Design review of the part built by this model. Coordinates are the model's own, in mm. Coordinates: 2 decimals unless noted, no trailing zeros. Loops run counter-clockwise (first coordinate to the right, second up) from the corner with the lowest first, then second, coordinate; pieces in that order, holes last. Notation, with made-up numbers: (-23.5, -27.5) -> (27.5, -27.5) arc R11 ccw to (27.5, -18.5) -> close; hole circle Ø9 at (0, 8.25). An arc over 180 degrees is marked (long way). Answer in a Markdown table with one row per item.
Autodesk Inventor part; units mm, degrees
ref_plane "Start plane" through (0, 0, -17.5) normal (0, 0, 1) x (1, 0, 0)
ref_plane "End plane" through (0, 0, 447.5) normal (0, 0, 1) x (1, 0, 0)
ref_plane "Work Plane4" through (17.5, 0, 447.5) normal (-0.7071, 0, 0.7071) x (0.7071, 0, 0.7071)
ref_plane "Start plane" through (0, 0, -17.5) normal (0, 0, 1) x (1, 0, 0)
ref_plane "End plane" through (0, 0, 447.5) normal (0, 0, 1) x (1, 0, 0)
sketch "Sketch" plane through (0, 0, 0) normal (0, 0, 1) x (1, 0, 0)
  line L0 (-17.5, -14.3) -> (-17.5, 14.3)
  line L1 (-14.3, 17.5) -> (14.3, 17.5)
  line L2 (17.5, 14.3) -> (17.5, -14.3)
  line L3 (14.3, -17.5) -> (-14.3, -17.5)
  arc A0 (-17.5, -14.3) -> (-14.3, -17.5) centre (-14.3, -14.3) ccw
  arc A1 (-14.3, 17.5) -> (-17.5, 14.3) centre (-14.3, 14.3) ccw
  arc A2 (17.5, 14.3) -> (14.3, 17.5) centre (14.3, 14.3) ccw
  arc A3 (14.3, -17.5) -> (17.5, -14.3) centre (14.3, -14.3) ccw
  arc A4 (-14.3, 15.9) -> (-15.9, 14.3) centre (-14.3, 14.3) ccw
  line L4 (-14.3, 15.9) -> (14.3, 15.9)
  arc A5 (15.9, 14.3) -> (14.3, 15.9) centre (14.3, 14.3) ccw
  line L5 (15.9, 14.3) -> (15.9, -14.3)
  arc A6 (14.3, -15.9) -> (15.9, -14.3) centre (14.3, -14.3) ccw
  line L6 (14.3, -15.9) -> (-14.3, -15.9)
  arc A7 (-15.9, -14.3) -> (-14.3, -15.9) centre (-14.3, -14.3) ccw
  line L7 (-15.9, -14.3) -> (-15.9, 14.3)
  line L8 (0, 25.4278) -> (0, -25.4278) construction
  line L9 (-25.4278, 0) -> (25.4278, 0) construction
  dimension "d7" = 3.2
  dimension "d10" = 35
  dimension "d11" = 35
  dimension "d12" = 1.6
  dimension "d15" = 17.5
  dimension "d16" = 17.5
extrude "Body" add sketch "Sketch" along normal up to surface (465 mm away) from surface at -17.5
sketch "Sketch3" plane through (0, 0, 0) normal (0, 0, 1) x (1, 0, 0)
  line L0 (0, 0) -> (10, 0)
ref_plane "Work Plane3" through (0, 0, 0) normal (0, -1, 0) x (1, 0, 0)
sketch "Sketch4" plane through (0, 0, 0) normal (0, -1, 0) x (1, 0, 0)
  line L0 (-2, -17.5) -> (12, -17.5)
  line L1 (-2, 447.5) -> (12, 447.5)
  dimension "d18" = 465
ref_plane "Work Plane4" through (17.5, 0, 447.5) normal (-0.7071, 0, 0.7071) x (0.7071, 0, 0.7071)
split "Split1" plane through (17.5, 0, 447.5) removes the side toward (-0.7071, 0, 0.7071)
ref_plane "Work Plane5" through (17.5, 0, -17.5) normal (-0.7071, 0, -0.7071) x (-0.7071, 0, 0.7071)
split "Split2" plane through (17.5, 0, -17.5) removes the side toward (-0.7071, 0, -0.7071)
ref_plane "Work Plane6" through (-730, 0, 215) normal (1, 0, 0) x (0, 0, -1)
ref_plane "Work Plane7" through (0, 0, 215) normal (1, 0, 0) x (0, 0, -1)
ref_plane "Work Plane8" through (-365, 0, 215) normal (1, 0, 0) x (0, 0, -1)
sketch "Sketch5" plane through (-365, 0, 215) normal (1, 0, 0) x (0, 0, -1)
  arc A0 (-17.5, -11.5) -> (-11.5, -17.5) centre (-11.5, -11.5) ccw
  line L0 (-17.5, -11.5) -> (-17.5, 11.5)
  arc A1 (-11.5, 17.5) -> (-17.5, 11.5) centre (-11.5, 11.5) ccw
  line L1 (-11.5, 17.5) -> (11.5, 17.5)
  arc A2 (17.5, 11.5) -> (11.5, 17.5) centre (11.5, 11.5) ccw
  line L2 (17.5, 11.5) -> (17.5, -11.5)
  arc A3 (11.5, -17.5) -> (17.5, -11.5) centre (11.5, -11.5) ccw
  line L3 (11.5, -17.5) -> (-11.5, -17.5)
  arc A4 (-11.5, 14.5) -> (-14.5, 11.5) centre (-11.5, 11.5) ccw
  line L4 (-11.5, 14.5) -> (11.5, 14.5)
  arc A5 (14.5, 11.5) -> (11.5, 14.5) centre (11.5, 11.5) ccw
  line L5 (14.5, 11.5) -> (14.5, -11.5)
  arc A6 (11.5, -14.5) -> (14.5, -11.5) centre (11.5, -11.5) ccw
  line L6 (11.5, -14.5) -> (-11.5, -14.5)
  arc A7 (-14.5, -11.5) -> (-11.5, -14.5) centre (-11.5, -11.5) ccw
  line L7 (-14.5, -11.5) -> (-14.5, 11.5)
extrude "Extrusion2" cut sketch "Sketch5" along normal up to surface (730 mm away) from surface at -365 contours L0 A1 L1 A2 L2 A3 L3 A0 | L4 A5 L5 A6 L6 A7 L7 A4
equation "\"d7\" = G_IR"
equation "\"d10\" = G_H"
equation "\"d11\" = G_W"
equation "\"d12\" = G_T"
equation "\"d15\" = 0.5 * d10"
equation "\"d16\" = 0.5 * d11"
equation "\"d3\" = G_L"
equation "\"G_W\" = 35"
equation "\"G_H\" = 35"
equation "\"G_T\" = 1.6"
equation "\"G_IR\" = 3.2"
equation "\"G_L\" = d18"
equation "\"G_OFFSET_START\" = 17.5"
equation "\"G_OFFSET_END\" = 17.5"
equation "\"d13\" = -G_OFFSET_START"
equation "\"d14\" = G_OFFSET_END + B_L"
properties part number "AS C350L0 35x35x3.0 SHS 00000050" material "Steel, Mild"
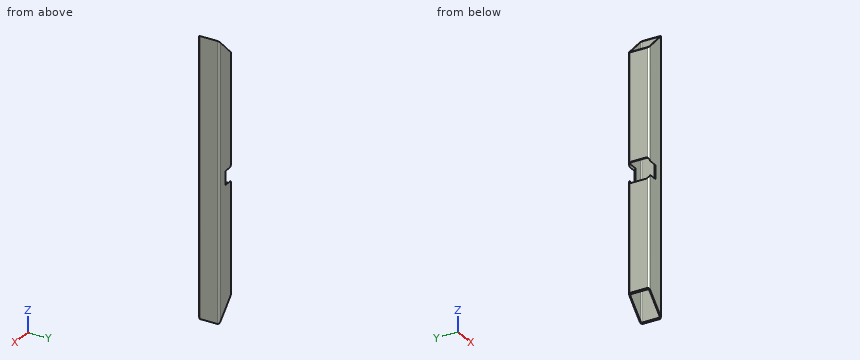
(1) Take a section at C-C on z = 144.5. Give the boundary of the cut face in (x, y).
Evaluation:
| item | result |
|---|---|
| outline | (-17.5, -14.3) arc R3.2 ccw to (-14.3, -17.5) -> (14.3, -17.5) arc R3.2 ccw to (17.5, -14.3) -> (17.5, 14.3) arc R3.2 ccw to (14.3, 17.5) -> (-14.3, 17.5) arc R3.2 ccw to (-17.5, 14.3) -> close; hole (-15.9, -14.3) arc R1.6 ccw to (-14.3, -15.9) -> (14.3, -15.9) arc R1.6 ccw to (15.9, -14.3) -> (15.9, 14.3) arc R1.6 ccw to (14.3, 15.9) -> (-14.3, 15.9) arc R1.6 ccw to (-15.9, 14.3) -> close |
(2) Take a section at A-A on x = 7.5. Give the boundary of the cut face in (y, z), and give its area (3 significant figures).
Evaluation:
| item | result |
|---|---|
| outline | (-17.5, -7.5) -> (-15.9, -7.5) -> (-15.9, 437.5) -> (-17.5, 437.5) -> close; (15.9, -7.5) -> (17.5, -7.5) -> (17.5, 437.5) -> (15.9, 437.5) -> close |
| area | 1,420 mm² |
(3) For pin 1 (10 mm diameter, centred on x = 13, y = 4.5, fed in from +Z); pin 2 (1.3 mm diameter, centred on y = -17, z = 207.5, fed in from -X); pin 3 (0.5 mm diameter, centred on x = -16.5, y = 5.5, fed in from -Z); pin 4 (0.5 mm diameter, centred on x = -16.5, y = -3, fed in from +Z), all flat-tipped, find the tip position at first contact; note any pin that passes through.
Evaluation:
| item | result |
|---|---|
| pin 1 | stops at z = 447.5 |
| pin 2 | stops at x = 0 |
| pin 3 | stops at z = 16.25 |
| pin 4 | stops at z = 413.75 |
(4) Take a section at B-B on y = -6. Give the boundary of the cut face in (x, z), and give its area (3 significant figures).
Evaluation:
| item | result |
|---|---|
| outline | (-17.5, 17.5) -> (-15.9, 15.9) -> (-15.9, 197.5) -> (-17.5, 197.5) -> close; (-17.5, 232.5) -> (-15.9, 232.5) -> (-15.9, 414.1) -> (-17.5, 412.5) -> close; (15.9, -15.9) -> (17.5, -17.5) -> (17.5, 447.5) -> (15.9, 445.9) -> close |
| area | 1,320 mm² |
(5) To check wall thickness, follow probe 1 along X at (y, z) = (5, 254); probe 2 along Z at (x, y) = (-16, -12). State the ranges of each line that lie inside material, in increasing order.
Evaluation:
| item | result |
|---|---|
| probe 1 | x = -17.5 to -15.9, 15.9 to 17.5 |
| probe 2 | z = 16 to 197.52, 232.48 to 414 |
